Part print with two shaded views. Sizes in mm from the minimum x, y, z corner. Give positions to 0.01 mm unless a question says otherwise; leave off trailing zeros. Write each loop counter-clockwise with the first axis right and the second up, starting at its lowest first coordinate (ties: lowest second). Pieces come first, ordered by that corner, then holes. Notation, with made-up numbers: (-14.75, 75.5) -> (-6.75, 75.5) arc R28 cw to (-6.75, 113.5) -> close; hole circle Ø2 at (54, 68). An arc over 180 degrees is marked (long way). Answer as a JSON object with one key per item and string values.
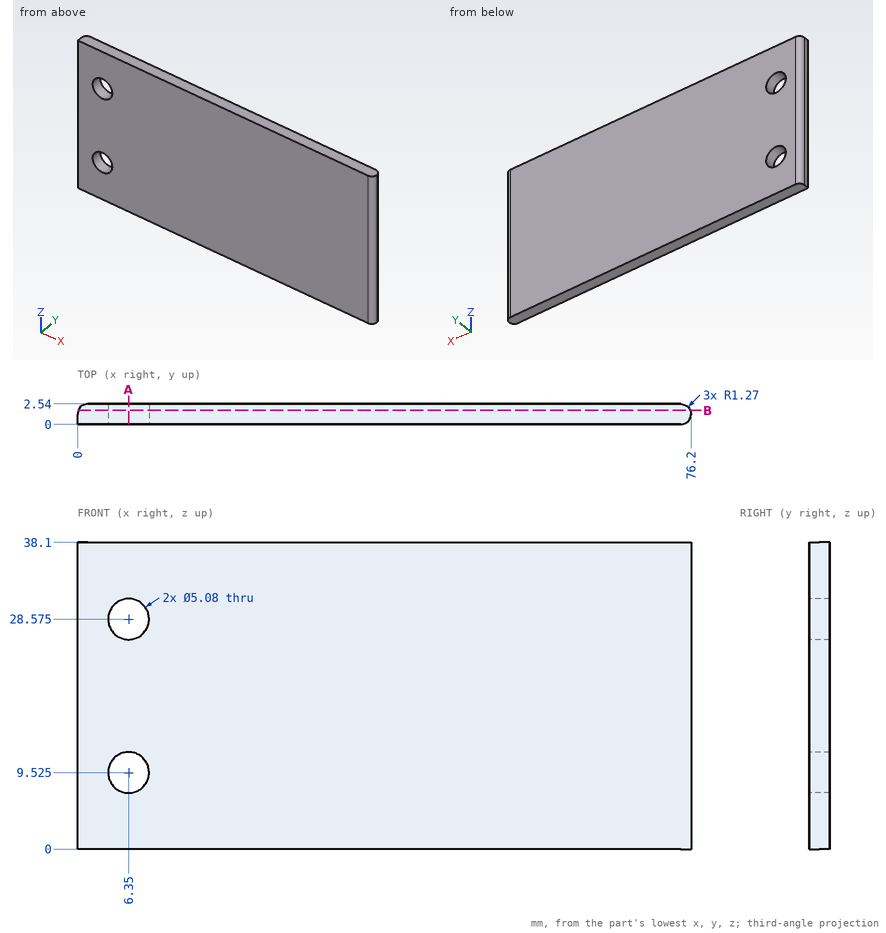
1) Slice it at A-A (x = 6.35). List the corners of the cut face in (y, z) (3 decimals), then the cut area to 3 significant figures.
Model answer:
{"outline": "(0, 0) -> (2.54, 0) -> (2.54, 6.985) -> (0, 6.985) -> close; (0, 12.065) -> (2.54, 12.065) -> (2.54, 26.035) -> (0, 26.035) -> close; (0, 31.115) -> (2.54, 31.115) -> (2.54, 38.1) -> (0, 38.1) -> close", "area": "71.0 mm2"}
2) Pin check, flat tip, straight feed: pin 1 (3 mm diameter, centred on x = 6.35, z = 28.575, fed in from -Y). Stop position of the tip, or through.
Model answer:
{"pin 1": "passes through"}
3) Slice it at B-B (y = 1.75). List the corners of the cut face in (x, z) (3 decimals).
Model answer:
{"outline": "(0.094, 0) -> (76.106, 0) -> (76.106, 38.1) -> (0.094, 38.1) -> close; hole circle Ø5.08 at (6.35, 9.525); hole circle Ø5.08 at (6.35, 28.575)"}
4) Wall check: probe 1 along Z at (x, y) = (6.35, 0.75) (3 decimals); probe 2 along X at (y, z) = (1.05, 29); probe 3 along Z at (x, y) = (8.5, 0.15). Give the ranges that are in metal, low to high.
Model answer:
{"probe 1": "z = 0 to 6.985, 12.065 to 26.035, 31.115 to 38.1", "probe 2": "x = 0 to 3.85, 8.85 to 76.18", "probe 3": "z = 0 to 8.17, 10.88 to 27.22, 29.93 to 38.1"}
